Autodesk Inventor part; units mm, degrees
ref_plane "Work Plane2" through (0, 25, 45) normal (0, 1, 0) x (1, 0, 0)
ref_plane "YZ Plane" through (0, 0, 0) normal (1, 0, 0) x (0, 1, 0)
ref_plane "XZ Plane" through (0, 0, 0) normal (0, 1, 0) x (-1, 0, 0)
sketch "Sketch1" plane through (0, 0, 0) normal (0, 0, 1) x (1, 0, 0)
  line L0 (0, 0) -> (40, 0)
  line L1 (40, 0) -> (40, 100)
  line L2 (40, 100) -> (0, 100)
  line L3 (0, 100) -> (0, 0)
  dimension "d0" = 40
  dimension "d1" = 100
extrude "Extrusion1" add sketch "Sketch1" along normal blind 45
sketch "Sketch2" plane through (0, 0, 0) normal (0, 0, -1) x (-1, 0, 0)
  line L0 (-40, 0) -> (-40, 100)
  line L1 (-40, 100) -> (10, 100)
  line L2 (10, 100) -> (10, 0)
  line L3 (10, 0) -> (-40, 0)
  line L4 (-40, 0) -> (-40, 100)
  point P0 (0, 0)
  dimension "d4" = 10
extrude "Extrusion2" add sketch "Sketch2" along normal blind 37.5
sketch "Sketch3" plane through (40, 0, 45) normal (1, 0, 0) x (0, 0, -1)
  line L0 (82.5, 100) -> (0, 100)
  line L1 (0, 0) -> (0, 100)
  line L2 (82.5, 0) -> (0, 0)
  line L3 (82.5, 100) -> (82.5, 0)
  line L4 (5, 5) -> (5, 95)
  line L5 (5, 95) -> (77.5, 95)
  line L6 (77.5, 95) -> (77.5, 5)
  line L7 (77.5, 5) -> (5, 5)
  point P0 (45, 0)
  dimension "d7" = 5
extrude "Extrusion3" cut sketch "Sketch3" against normal blind 35 contours L4 L5 L6 L7
sketch "Sketch4" plane through (5, 0, 45) normal (1, 0, 0) x (0, 0, -1)
  line L0 (45, 100) -> (45, 0)
  line L1 (45, 100) -> (82.5, 100)
  line L2 (82.5, 0) -> (82.5, 100)
  line L3 (45, 0) -> (82.5, 0)
  line L4 (50, 5) -> (50, 95)
  line L5 (50, 95) -> (77.5, 95)
  line L6 (77.5, 95) -> (77.5, 5)
  line L7 (77.5, 5) -> (50, 5)
  point P0 (45, 0)
  dimension "d10" = 5
extrude "Extrusion4" cut sketch "Sketch4" against normal blind 10 contours L4 L5 L6 L7
sketch "Sketch5" plane through (0, 0, 45) normal (0, -1, 0) x (1, 0, 0)
  line L0 (0, 0) -> (40, 0)
  line L1 (0, -45) -> (0, 0)
  line L2 (-10, -45) -> (0, -45)
  line L3 (-10, -45) -> (-10, -82.5)
  line L4 (40, -82.5) -> (-10, -82.5)
  line L5 (40, -77.5) -> (-5, -77.5)
  line L6 (-5, -77.5) -> (-5, -50)
  line L7 (-5, -50) -> (5, -50)
  line L8 (5, -50) -> (5, -5)
  line L9 (5, -5) -> (40, -5)
  line L10 (40, -77.5) -> (40, -5)
  line L11 (40, -82.5) -> (40, 0)
  dimension "d13" = 5
extrude "Extrusion5" cut sketch "Sketch5" against normal through all contours L10 L5 L6 L7 L8 L9
sketch "Sketch6" plane through (0, 100, 45) normal (0, 1, 0) x (1, 0, 0)
  line L0 (0, 45) -> (0, 0)
  line L1 (0, 0) -> (40, 0)
  line L2 (40, 0) -> (40, 10)
  line L3 (40, 10) -> (0, 10)
  line L4 (0, 10) -> (0, 0)
  dimension "d16" = 40
  dimension "d17" = 10
extrude "Extrusion6" add sketch "Sketch6" against normal blind 100
sketch "Sketch8" plane through (40, 100, 35) normal (0, 0, -1) x (-1, 0, 0)
  line L0 (35, 0) -> (35, -100)
  line L1 (0, 0) -> (35, 0)
  line L2 (0, 0) -> (0, -100)
  line L3 (35, -100) -> (0, -100)
  line L4 (35, -105) -> (0, -105)
  line L5 (0, -105) -> (0, 5)
  line L6 (0, 5) -> (35, 5)
  line L7 (35, 5) -> (35, -105)
  point P0 (40, -100)
  dimension "d20" = 5
  dimension "d21" = 5
extrude "Extrusion7" add sketch "Sketch8" along normal blind 5
sketch "Sketch10" plane through (5, 0, -5) normal (0, 0, -1) x (-1, 0, 0)
  line L0 (0, 0) -> (0, 100)
  line L1 (10, 0) -> (0, 0)
  line L2 (10, 0) -> (10, 100)
  line L3 (0, 100) -> (10, 100)
  line L4 (-35, -5) -> (0, -5)
  line L5 (10, 0) -> (0, 0)
  line L6 (0, 0) -> (0, -5)
  line L7 (0, -5) -> (10, -5)
  line L8 (10, -5) -> (10, 0)
  line L9 (0, 105) -> (0, 100)
  line L10 (10, 100) -> (0, 100)
  line L11 (0, 100) -> (0, 105)
  line L12 (0, 105) -> (10, 105)
  line L13 (10, 105) -> (10, 100)
  point P0 (5, 0)
extrude "Extrusion8" add sketch "Sketch10" along normal blind 5
sketch "Sketch25" plane through (5, 0, 45) normal (1, 0, 0) x (0, 0, -1)
  circle A0 centre (32.5, 25) radius 10
  circle A1 centre (32.5, 25) radius 2.5
  line L0 (50, 0) -> (15, 0)
  line L1 (15, 105) -> (15, -5)
  circle A2 centre (66.25, 25) radius 2.5
  circle A3 centre (66.25, 25) radius 10
  line L2 (77.5, 0) -> (55, 0)
  point P0 (32.5, 0)
  point P1 (15, 55)
  point P2 (15, 25)
  point P3 (66.25, 0)
  dimension "d89" = 20
  dimension "d90" = 5
  dimension "d93" = 5
  dimension "d94" = 20
extrude "Extrusion22" add sketch "Sketch25" along normal blind 35 contours A3
sketch "Sketch26" plane through (-5, 0, 45) normal (1, 0, 0) x (0, 0, -1)
  circle A0 centre (66.25, 25) radius 10
  circle A1 centre (66.25, 25) radius 2.5
  point P0 (45, 0)
extrude "Extrusion23" add sketch "Sketch26" along normal blind 10
sketch "Sketch27" plane through (5, 0, 45) normal (1, 0, 0) x (0, 0, -1)
  circle A0 centre (54, 80) radius 10
  circle A1 centre (54, 80) radius 5
  line L0 (15, 105) -> (15, -5)
  line L1 (15, 100) -> (50, 100)
  point P0 (45, 0)
  dimension "d98" = 20
  dimension "d99" = 10
  dimension "d100" = 39
  dimension "d101" = 20
extrude "Extrusion24" add sketch "Sketch27" against normal blind 10
sketch "Sketch30" plane through (40, 0, 45) normal (1, 0, 0) x (0, 0, -1)
  line L0 (10, 0) -> (0, 0)
  line L1 (15, -5) -> (15, 0)
  line L2 (10, 0) -> (15, 0)
  line L3 (15, 0) -> (15, -5)
  line L4 (15, -5) -> (10, -5)
  line L5 (10, -5) -> (10, 0)
  point P0 (45, 0)
extrude "Extrusion27" cut sketch "Sketch30" against normal through all
sketch "Sketch31" plane through (40, 100, 30) normal (0, 0, -1) x (-1, 0, 0)
  line L0 (40, -100) -> (0, -100)
  line L1 (0, -100) -> (0, 0)
  line L2 (0, 0) -> (40, 0)
  line L3 (40, 0) -> (40, -100)
  line L4 (10, -95) -> (25, -95)
  line L5 (25, -95) -> (25, -85)
  line L6 (25, -85) -> (10, -85)
  line L7 (10, -85) -> (10, -95)
  line L8 (35, 0) -> (35, -100)
  dimension "d110" = 15
  dimension "d111" = 10
  dimension "d112" = 10
  dimension "d113" = 5
extrude "Extrusion28" cut sketch "Sketch31" against normal blind 5 contours L7 L6 L5 L4
fillet "Fillet1" radius 2 4 edges at (15, 10, 30) (30, 10, 30) (15, 10, 35) (30, 10, 35)
sketch "Sketch32" plane through (0, 0, 45) normal (0, -1, 0) x (1, 0, 0)
  line L0 (2, -11) -> (33, -11) construction
  line L1 (33, -11) -> (33, -42) construction
  line L2 (33, -42) -> (2, -42) construction
  line L3 (2, -42) -> (2, -11) construction
  line L4 (40, -82.5) -> (-10, -82.5) construction
  line L5 (40, 0) -> (40, -15) construction
  circle A0 centre (33, -11) radius 2.5
  point P0 (0, -45)
  dimension "d117" = 31
  dimension "d118" = 31
  dimension "d119" = 40.5
  dimension "d120" = 7
  dimension "d121" = 5
extrude "Extrusion29" cut sketch "Sketch32" against normal blind 5
sketch "Sketch33" plane through (0, 100, 45) normal (0, 1, 0) x (1, 0, 0)
  circle A0 centre (17.5, 26.5) radius 6
  circle A1 centre (17.5, 26.5) radius 9 construction
  line L0 (26.5, 26.5) -> (26.5, 15)
  line L1 (8.5, 15) -> (26.5, 15)
  line L2 (17.5, 35.5) -> (5, 35.5)
  line L3 (5, 15) -> (5, 50)
  line L4 (5, 35.5) -> (5, 15)
  line L5 (40, 15) -> (5, 15)
  line L6 (5, 15) -> (40, 15)
  line L7 (8.5, 15) -> (5, 15)
  arc A2 (26.5, 26.5) -> (17.5, 35.5) centre (17.5, 26.5) ccw
  point P0 (0, 45)
  dimension "d125" = 12
  dimension "d127" = 18
  dimension "d130" = 12.5
  dimension "d131" = 11.5
extrude "Extrusion32" add sketch "Sketch33" against normal blind 10
sketch "Sketch35" plane through (5, 0, 45) normal (1, 0, 0) x (0, 0, -1)
  circle A0 centre (54, 80) radius 10
  circle A1 centre (54, 80) radius 23
  point P0 (45, 0)
  dimension "d136" = 46
extrude "Extrusion33" cut sketch "Sketch35" along normal through all
ref_plane "Work Plane2" through (0, 25, 45) normal (0, 1, 0) x (1, 0, 0)
sketch "Sketch36" plane through (0, 25, 45) normal (0, 1, 0) x (1, 0, 0)
  line L0 (5, 50) -> (5, 15)
  line L1 (5, 15) -> (40, 15)
  circle A0 centre (17.5, 26.5) radius 6 construction
  circle A1 centre (17.5, 26.5) radius 9.5
  circle A2 centre (17.5, 26.5) radius 14 construction
  line L2 (31.5, 26.5) -> (31.5, 15)
  line L3 (31.5, 15) -> (5, 15)
  line L4 (5, 40.5) -> (5, 15)
  line L5 (17.5, 40.5) -> (5, 40.5)
  arc A3 (31.5, 26.5) -> (17.5, 40.5) centre (17.5, 26.5) ccw
  point P0 (0, 45)
  dimension "d140" = 19
  dimension "d141" = 28
extrude "Extrusion34" add sketch "Sketch36" along normal blind 10
sketch "Sketch37" plane through (5, 0, 45) normal (1, 0, 0) x (0, 0, -1)
  arc A0 (55, 75.101) -> (55, 84.899) centre (54, 80) ccw
  circle A1 centre (54, 80) radius 5
  point P0 (45, 0)
extrude "Extrusion35" cut sketch "Sketch37" against normal blind 10
sketch "Sketch38" plane through (0, 0, 45) normal (-1, 0, 0) x (0, 0, 1)
  arc A0 (-45, 75.6411) -> (-45, 84.3589) centre (-54, 80) ccw
  line L0 (-45, 75.6411) -> (-45, 0)
  line L1 (-45, 0) -> (0, 0)
  line L2 (0, 100) -> (0, 0)
  line L3 (-45, 100) -> (0, 100)
  line L4 (-45, 100) -> (-45, 84.3589)
  line L5 (-45, 0) -> (0, 0)
  line L6 (0, 0) -> (0, 100)
  line L7 (0, 100) -> (-45, 100)
  line L8 (-45, 100) -> (-45, 0)
extrude "Extrusion36" cut sketch "Sketch38" along normal through all
sketch "Sketch39" plane through (-10, 0, 0) normal (-1, 0, 0) x (0, 0, 1)
  circle A0 centre (-9, 80) radius 5
  circle A1 centre (-9, 80) radius 2.5
  point P0 (0, 0)
  dimension "d148" = 5
extrude "Extrusion37" cut sketch "Sketch39" against normal through all contours A1
properties part number "BA003" material "ABS Plastic"
Can you work these out from the model? Positions are in its coordinate system, mm. A direction names the side the tool comes from. Round coordinates to 2 decimals unless told otherwise and drop trailing zeros. Loops run counter-clockwise (first coordinate to the right, second up) from the corner with the lowest first, then second, coordinate; pieces in that order, holes last.
Item 1: Which directions (+Z, -Z, +X, -X, +Y, -Y) give clear straight access to the entire face, cutting with the end or side of a thin tool? Please do faces 4 (the flat face through (31.5, 30, 24)), 5 (the flat face through (13, 90, 23)), 6 (the flat face through (11, 97, 9.5)), 7 (the flat face through (-5, 102, -7)), 8 (the flat face through (22, 15, 32)).
Item 2: Suppose I cut it at B-B, the plane x = -2.5. Write out the boundary of the cut face in (y, z), then the cut area to 3 significant figures.
Item 3: Will these pins go through, and if not, where does the flat tip stop? pin 1 Ø2 at (x, y) = (-4, 80.5) entering from +Z; pin 2 Ø11 at (y, z) = (29, 21.5) entering from +X; pin 3 Ø3 at (x, z) = (25, 19.5) entering from -Y.
Item 4: Please list where these lines run through material, in increasing order: L1, parallel to Z at x = 33, y = 1; L2, parallel to Z at x = 17, y = 95; L3, parallel to Z at x = 17, y = 57.
Item 5: Suppose I cut it at C-C, the plane z = 26. Write out the boundary of the cut face in (x, y), then the cut area to 3 significant figures.
Item 6: Suppose I cut it at D-D, the plane z = -21.25. Write out the boundary of the cut face in (x, y), then the cut area to 4 significant figures.
Item 7: Suppose I cut it at A-A, the plane y = 68.5. Write out the boundary of the cut face in (x, z), then the cut area to 3 significant figures.
Item 8: If we mould it in two halves opening along Z, with no side actions, what happens to faces 1 (the flat face through (20, 51, 45)), 2 (the cylindrical face through (9.96, 29.93, 12.72)), 3 (the flat face through (0, 105, -7))? For each: +Z half, -Z half, draft (parallel to the pull), parting line (faces both ways), or undercut.
Reported:
1. face 4: +X, +Y, -Y
1. face 5: +X
1. face 6: +X, +Y
1. face 7: +Z, -Z, -X, +Y
1. face 8: none
2. outline: (-5, -10) - (70.05, -10) arc R10 ccw to (89.95, -10) - (105, -10) - (105, -5) - (100, -5) - (100, 0) - (0, 0) - (0, -5) - (-5, -5) - close; (0, -37.5) - (100, -37.5) - (100, -32.5) - (0, -32.5) - close; circle Ø20 at (25, -21.25); hole circle Ø5 at (25, -21.25); hole circle Ø10 at (80, -9)
2. area: 1,900 mm2
3. pin 1: stops at z = 0
3. pin 2: stops at x = 31.5
3. pin 3: stops at y = 90
4. L1: z = -37.5 to -32.5, 30 to 31.5, 36.5 to 45
4. L2: z = -37.5 to -32.5, 9.5 to 12.52, 24.48 to 45
4. L3: z = -37.5 to -32.5, 30 to 45
5. outline: (0, 0) - (5, 0) - (5, 25) - (11.67, 25) - (11.67, 35) - (5, 35) - (5, 90) - (26.5, 90) - (26.5, 100) - (0, 100) - close; (23.33, 25) - (31.5, 25) - (31.5, 35) - (23.33, 35) - close
5. area: 863 mm2
6. outline: (-10, 0) - (-5, 0) - (-5, 15) - (40, 15) - (40, 22.5) - (-5, 22.5) - (-5, 27.5) - (40, 27.5) - (40, 35) - (-5, 35) - (-5, 100) - (-10, 100) - close
6. area: 1,175 mm2
7. outline: (-10, -37.5) - (40, -37.5) - (40, -32.5) - (-5, -32.5) - (-5, -10) - (5, -10) - (5, 30) - (40, 30) - (40, 45) - (0, 45) - (0, 0) - (-10, 0) - close
7. area: 1,260 mm2
8. face 1: +Z half
8. face 2: undercut
8. face 3: draft
